Could you check a few things on this drawing? It's one solid part, dimensions in mm from its lowest x, y, z. Give positions to 0.01 mm unless a question says otherwise; leave off trailing zeros. Order: outer loops, then holes, each group sorted by start corner. A loop starts at its lowest first (then second) coordinate and runs counter-clockwise, first axis right, second up. Notation, with made-up numbers: M 50,40.25 L 104,40.25 A15 cw 104,49.25 Z; hole C 82.5,68 d3. An arc over 180 degrees is marked long. Use one line per item in the form item = value. Start each with the question number.
1. We'd pull the mould along Y, two halves only. Please class the marked faces 1 and 2: +Y half, -Y half, draft (parallel to the pull), parting line (faces both ways), or undercut.
2. I want a section at B-B, the plane y = 12.5. List the corners of the cut face in (x, z) for me.
3. I need wall thicknesses on L1, parallel to Z at x = 11.5, y = 11.25; L2, parallel to Z at x = 8, y = 17.25; L3, parallel to X at y = 6.5, z = 14. Which ranges of each line are inside material? Lowest first, please.
4. Will these pins go through, and if not, where does the flat tip stop? P1, Ø10, axis at x = 10.5, z = 13, coming from the +Y side; P2, Ø6, axis at x = 15, z = 12.5, coming from the +Y side; P3, Ø1, axis at x = 14.5, y = 7.5, coming from the +Z side; P4, Ø3.5, axis at y = 8, z = 4, coming from the -X side.
5. I want a section at C-C, the plane z = 9.5. List the corners of the cut face in (x, y) for me, and give its area (3 significant figures).
6. I want a section at D-D, the plane y = 15.5. List the corners of the cut face in (x, z) for me.
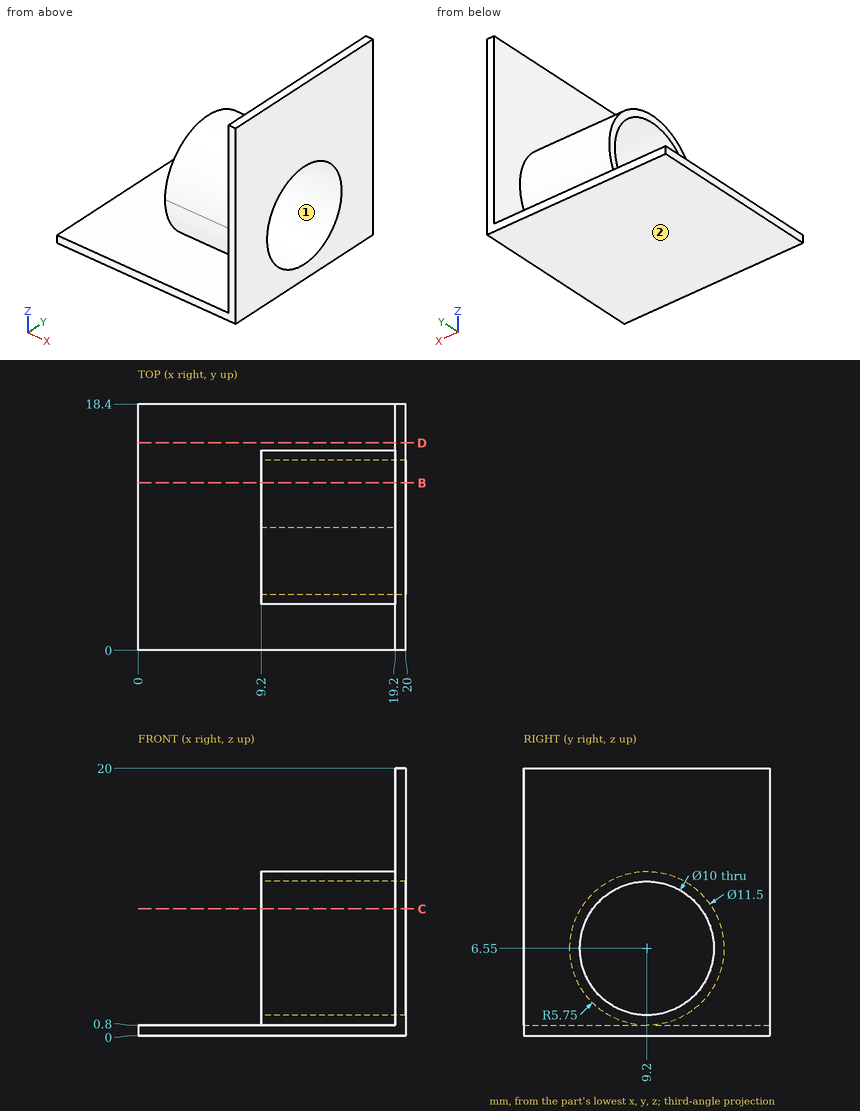
Check result:
q1.face_1 = undercut
q1.face_2 = draft
q2.outline = M 0,0 L 20,0 L 20,2.79 L 9.2,2.79 L 9.2,1.84 L 19.2,1.84 L 19.2,0.8 L 0,0.8 Z; M 9.2,10.31 L 20,10.31 L 20,20 L 19.2,20 L 19.2,11.26 L 9.2,11.26 Z
q3.L1 = 0 to 0.8, 1.18 to 1.99, 11.11 to 11.92
q3.L2 = 0 to 0.8
q3.L3 = 19.2 to 20
q4.P1 = 14.76
q4.P2 = 14.14
q4.P3 = 12.17
q4.P4 = through
q5.outline = M 9.2,4.26 L 19.2,4.26 L 19.2,0 L 20,0 L 20,5.16 L 9.2,5.16 Z; M 9.2,13.24 L 20,13.24 L 20,18.4 L 19.2,18.4 L 19.2,14.14 L 9.2,14.14 Z
q5.area = 26.2 mm2
q6.outline = M 0,0 L 20,0 L 20,20 L 19.2,20 L 19.2,0.8 L 0,0.8 Z
